```python
from build123d import *

# Parameters (mm, degrees)
SKETCH_W     = 25.4
SKETCH_H     = 25.4
SKETCH_R     = 2.6035
PAD_DEPTH    = 25.4
POCKET_DEPTH = 25.401
FILLET002_R  = 2


with BuildPart() as part:
    # Sketch → Pad (new body)
    with BuildSketch(Plane.XY):
        Rectangle(SKETCH_W, SKETCH_H)
        Circle(SKETCH_R, mode=Mode.SUBTRACT)
    extrude(amount=PAD_DEPTH)

    # Sketch001 (on Face7 of Pad) → Pocket (cut, through all)
    with BuildSketch(Plane.XY.offset(25.4)):
        Polygon((-3.2512, 4.5212), (3.2512, 4.5212), (9.2456, 10.5156), (3.2512, 10.5156), (3.2512, 12.7), (-3.2512, 12.7), (-3.2512, 10.5156), (-9.2456, 10.5156), align=None)
        Polygon((4.5212, 3.2512), (4.5212, -3.2512), (10.5156, -9.2456), (10.5156, -3.2512), (12.7, -3.2512), (12.7, 3.2512), (10.5156, 3.2512), (10.5156, 9.2456), align=None)
        Polygon((-3.2512, -4.5212), (3.2512, -4.5212), (9.2456, -10.5156), (3.2512, -10.5156), (3.2512, -12.7), (-3.2512, -12.7), (-3.2512, -10.5156), (-9.2456, -10.5156), align=None)
        Polygon((-4.5212, 3.2512), (-4.5212, -3.2512), (-10.5156, -9.2456), (-10.5156, -3.2512), (-12.7, -3.2512), (-12.7, 3.2512), (-10.5156, 3.2512), (-10.5156, 9.2456), align=None)
    extrude(amount=-POCKET_DEPTH, mode=Mode.SUBTRACT)

    # Fillet002
    fillet002_edges = [part.edges().sort_by_distance(p)[0] for p in [
        (12.7, -12.7, 12.7),
        (12.7, 12.7, 12.7),
        (-12.7, 12.7, 12.7),
        (-12.7, -12.7, 12.7),
    ]]
    fillet(fillet002_edges, radius=FILLET002_R)


solid = part.part
```
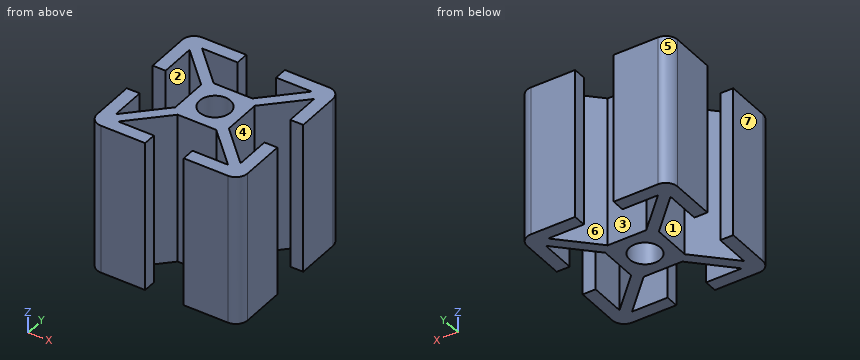
Design review of the part built by this model. Coordinates are the model's own, in mm. Face numbers are marked on the shaded views. A direction names the side the tool comes from. Give positions to 0.01 mm unless a question says otherwise; leave off trailing zeros. Write each loop counter-clockwise with the first axis right and the second up, starting at its lowest first coordinate (ties: lowest second). Pieces come first, ordered by that corner, then holes. Notation, with made-up numbers: (74, 80.5) - (124, 80.5) arc R9 ccw to (124, 97.5) - close; hole circle Ø8 at (74, 38). An arc over 180 degrees is marked (long way). Return JSON: item names as keys, results as strings. Group by question number.
(1) We need section A-A, the plane y = 0. Give the boundary of the cut face in (x, z), then the cut area to 3 significant figures.
(2) We need section C-C, the plane y = 5.25. Give the boundary of the cut face in (x, z).
(3) Machinability: for the marked faces 1, 2, 3 and 4, which of the approach directions +Z, -Z, +X, -X, +Y, -Y give a long, thin tool a straight path to every point of the face, cutting with its end or side? Answer none if there is none.
(4) Insertion check: pin 1 (1.1 mm diameter, centred on y = 12, z = 15, fed in from +X); pin 2 (1.1 mm diameter, centred on x = 11.5, z = 16.5, fed in from +Y); pin 3 (1.1 mm diameter, centred on x = 12, z = 10, fed in from -Y). Each pin has a flat end and moves straight along its axis. Give the tip position at first contact, or say it passes through.
(5) To check wall thickness, follow probe 1 along Y at (x, z) = (0, 9); probe 2 along Y at (x, z) = (10.75, 4.5); probe 3 along Y at (x, z) = (-8, 2). State the ranges of each line that lie inside material, in increasing order.
(6) Mouldability with a two-part tool opening along Y and no side actions: class the marked faces 5, 6 and 7 as +Y half, -Y half, draft (parallel to the pull), parting line (faces both ways), or undercut.
Reported:
{
 "1": {"outline": "(-4.52, 0) - (-2.6, 0) - (-2.6, 25.4) - (-4.52, 25.4) - close; (2.6, 0) - (4.52, 0) - (4.52, 25.4) - (2.6, 25.4) - close", "area": "97.4 mm2"},
 "2": {"outline": "(-12.7, 0) - (-10.52, 0) - (-10.52, 25.4) - (-12.7, 25.4) - close; (-6.52, 0) - (-3.98, 0) - (-3.98, 25.4) - (-6.52, 25.4) - close; (3.98, 0) - (6.52, 0) - (6.52, 25.4) - (3.98, 25.4) - close; (10.52, 0) - (12.7, 0) - (12.7, 25.4) - (10.52, 25.4) - close"},
 "3": {"face 1": "+Z, -Z, -X", "face 2": "+Z, -Z", "face 3": "+Z, -Z, +Y", "face 4": "+Z, -Z, +X"},
 "4": {"pin 1": "stops at x = 12.55", "pin 2": "stops at y = 12.68", "pin 3": "stops at y = -12.55"},
 "5": {"probe 1": "y = -4.52 to -2.6, 2.6 to 4.52", "probe 2": "y = -12.7 to -3.25, 3.25 to 12.7", "probe 3": "y = -12.7 to -10.52, -9.27 to -6.73, 6.73 to 9.27, 10.52 to 12.7"},
 "6": {"face 5": "+Y half", "face 6": "undercut", "face 7": "draft"}
}
